from build123d import *

# Parameters (mm, degrees)
PAD_DEPTH       = 0.4
SKETCH001_R     = 2
POCKET_DEPTH    = 5
PAD001_DEPTH    = 6.15
POCKET001_DEPTH = 6.551
FILLET_R        = 0.5
FILLET001_R     = 0.39
FILLET002_R     = 0.9


with BuildPart() as part:
    # Sketch → Pad (new body)
    with BuildSketch(Plane.XY):
        with BuildLine():
            Line((-13.4, 6.275), (13.4, 6.275))
            ThreePointArc((15.4, 4.275), (14.814214, 5.689214), (13.4, 6.275))
            Line((15.4, 4.275), (15.4, -4.275))
            ThreePointArc((13.4, -6.275), (14.814214, -5.689214), (15.4, -4.275))
            Line((13.4, -6.275), (-13.4, -6.275))
            ThreePointArc((-15.4, -4.275), (-14.814214, -5.689214), (-13.4, -6.275))
            Line((-15.4, -4.275), (-15.4, 4.275))
            ThreePointArc((-13.4, 6.275), (-14.814214, 5.689214), (-15.4, 4.275))
        make_face()
    extrude(amount=PAD_DEPTH)

    # Sketch001 (on Face10 of Pad) → Pocket (cut)
    with BuildSketch(Plane.XY.offset(0.4)):
        with Locations((-12.495, 0)):
            Circle(SKETCH001_R)
        with Locations((12.495, 0)):
            Circle(SKETCH001_R)
    extrude(amount=-POCKET_DEPTH, mode=Mode.SUBTRACT)

    # Sketch002 (on Face5 of Pocket) → Pad001 (join)
    with BuildSketch(Plane.XY.offset(0.4)):
        with BuildLine():
            Line((-5.475, 3.935), (5.475, 3.935))
            ThreePointArc((7.981365, 0.948231), (7.424529, 3.025959), (5.475, 3.935))
            Line((7.981365, 0.948231), (7.491365, -1.831769))
            ThreePointArc((4.985, -3.935), (6.620959, -3.339529), (7.491365, -1.831769))
            Line((4.985, -3.935), (-4.985, -3.935))
            ThreePointArc((-7.491365, -1.831769), (-6.620959, -3.339529), (-4.985, -3.935))
            Line((-7.491365, -1.831769), (-7.981365, 0.948231))
            ThreePointArc((-5.475, 3.935), (-7.424529, 3.025959), (-7.981365, 0.948231))
        make_face()
    extrude(amount=PAD001_DEPTH)

    # Sketch003 (on Face21 of Pad001) → Pocket001 (cut, through all)
    with BuildSketch(Plane.XY.offset(6.55)):
        with BuildLine():
            Line((-5.475, 3.535), (5.475, 3.535))
            ThreePointArc((7.587437, 1.017664), (7.11812, 2.768834), (5.475, 3.535))
            Line((7.587437, 1.017664), (7.097437, -1.762336))
            ThreePointArc((4.985, -3.535), (6.363834, -3.03312), (7.097437, -1.762336))
            Line((4.985, -3.535), (-4.985, -3.535))
            ThreePointArc((-7.097437, -1.762336), (-6.363834, -3.03312), (-4.985, -3.535))
            Line((-7.097437, -1.762336), (-7.587437, 1.017664))
            ThreePointArc((-5.475, 3.535), (-7.11812, 2.768834), (-7.587437, 1.017664))
        make_face()
    extrude(amount=-POCKET001_DEPTH, mode=Mode.SUBTRACT)

    # Fillet
    fillet_edges = [part.edges().sort_by_distance(p)[0] for p in [
        (0, -3.935, 0.4),
    ]]
    fillet(fillet_edges, radius=FILLET_R)

    # Fillet001
    fillet001_edges = [part.edges().sort_by_distance(p)[0] for p in [
        (-6.620959, -3.339529, 6.55),
    ]]
    fillet(fillet001_edges, radius=FILLET001_R)

    # Fillet002
    fillet002_edges = [part.edges().sort_by_distance(p)[0] for p in [
        (0, 3.535, 0),
    ]]
    fillet(fillet002_edges, radius=FILLET002_R)


solid = part.part
CAD build for the part. Positions are in the model's coordinates, mm. A direction names the side the tool comes from. Coordinates: 2 decimals unless noted, no trailing zeros. Write each loop counter-clockwise with the first axis right and the second up, starting at its lowest first coordinate (ties: lowest second). Pieces come first, ordered by that corner, then holes. Notation, with made-up numbers: (54, 69.25) - (101, 69.25) arc R27 ccw to (101, 90.25) - close; hole circle Ø1 at (5.5, 34). An arc over 180 degrees is marked (long way). Use a Markdown table: item, result. Add a question column.
Item 1: Flat gauge pins, fed straight in: pin 1 (2 mm diameter, centred on y = 1, z = 3.5, fed in from +X); pin 2 (3 mm diameter, centred on y = 0, z = 1, fed in from -X); pin 3 (1.5 mm diameter, centred on x = 7, z = 4, fed in from -Y); pin 4 (3 mm diameter, centred on x = -2, z = 4, fed in from +Y) (3 decimals). Where does each tip first touch, or does it go through?
Item 2: Mould opens along Y. For faces 1 (the face through (7.135, 2.749, 3.765)), 2 (the face through (0, 6, 0)), 3 (the face through (-14.799, 5.705, 0.197)) say: pulls with the +Y half, pulls with the -Y half, needs draft (parallel to the pull), parting line crosses it, or undercut.
Item 3: Drill centre lines: L1, parallel to Y at x = 1, z = 3.25 (3 decimals); L2, parallel to X at y = -3.25, z = 5.5; L3, parallel to X at y = -2.5, z = 6. Where is each one in solid material? Low to high. Write a range as from..to.
Item 4: Band-saw the part on D-D, the plane y = -5.25. Give the cut face in (x, z).
Item 5: 3-axis set-ups, long thin cutter, end or side, ignore diameter. For faces 4 (the face through (0, -3.935, 3)), 5 (the face through (-7.733, -0.461, 3.493)), 6 (the face through (-0.08, 3.79, 0.27)), 7 (the face through (7.74, -0.42, 3.49)), 8 (the face through (0, -3.535, 4)): which of +Z, -Z, +X, -X, +Y, -Y reach the whole face in a straight line?
Item 6: Band-saw the part on B-B, the plane z = 2.25. Give the cut face in (x, y) (3 decimals).
Item 7: Band-saw the part on C-C, the plane y = 0. Give the number of separate pieces and of enclosed holes in the cut face, and give its area (3 significant figures).
Item 8: Band-saw the part on A-A, the plane x = 1.5. Give the cut face in (y, z) (3 decimals), and give its area (3 significant figures).
Numbers:
| question | item | result |
|---|---|---|
| 1 | pin 1 | x = 8.02 |
| 1 | pin 2 | x = -15.4 |
| 1 | pin 3 | y = -3.6 |
| 1 | pin 4 | y = 3.935 |
| 2 | face 1 | undercut |
| 2 | face 2 | needs draft |
| 2 | face 3 | pulls with the +Y half |
| 3 | L1 | -3.935..-3.535, 3.535..3.935 |
| 3 | L2 | -6.72..-6.05, 6.05..6.72 |
| 3 | L3 | -7.28..-6.82, 6.82..7.28 |
| 4 | outline | (-15.15, 0) - (15.15, 0) - (15.15, 0.4) - (-15.15, 0.4) - close |
| 5 | face 4 | +Z, +X, -X, -Y |
| 5 | face 5 | +Z, -X, -Y |
| 5 | face 6 | -Z |
| 5 | face 7 | +Z, +X, -Y |
| 5 | face 8 | +Z, -Z |
| 6 | outline | (-7.981, 0.948) - (-7.491, -1.832) arc R2.545 ccw to (-4.985, -3.935) - (4.985, -3.935) arc R2.545 ccw to (7.491, -1.832) - (7.981, 0.948) arc R2.545 ccw to (5.475, 3.935) - (-5.475, 3.935) arc R2.545 ccw to start; hole (-7.587, 1.018) - (-7.097, -1.762) arc R2.145 ccw to (-4.985, -3.535) - (4.985, -3.535) arc R2.145 ccw to (7.097, -1.762) - (7.587, 1.018) arc R2.145 ccw to (5.475, 3.535) - (-5.475, 3.535) arc R2.145 ccw to start |
| 7 | separate pieces | 4 |
| 7 | enclosed holes | 0 |
| 7 | area | 7.88 mm2 |
| 8 | outline | (-6.275, 0) - (-4.435, 0) arc R0.9 ccw to (-3.535, 0.9) - (-3.535, 6.55) - (-3.545, 6.55) arc R0.39 ccw to (-3.935, 6.16) - (-3.935, 0.9) arc R0.5 cw to (-4.435, 0.4) - (-6.275, 0.4) - close; (3.535, 0.9) arc R0.9 ccw to (4.435, 0) - (6.275, 0) - (6.275, 0.4) - (4.435, 0.4) arc R0.5 cw to (3.935, 0.9) - (3.935, 6.16) arc R0.39 ccw to (3.545, 6.55) - (3.535, 6.55) - close |
| 8 | area | 6.81 mm2 |
